```python
from build123d import *

# Parameters (mm, degrees)
BOSS_EXTRUDE1_DEPTH = 3.175
CUT_EXTRUDE1_REACH  = 5.175


with BuildPart() as part:
    # Sketch1 → Boss-Extrude1 (new body)
    with BuildSketch(Plane(origin=(0, 0, 0), x_dir=(0, 0, -1), z_dir=(1, 0, 0))):
        Polygon((0, 0), (-837.664111915, 0), (-1066.8, -396.875), (-1066.8, -800.1), (0, -800.1), align=None)
    extrude(amount=BOSS_EXTRUDE1_DEPTH)

    # Sketch2 → Cut-Extrude1 (cut, up to next)
    with BuildSketch(Plane(origin=(3.175, 0, 0), x_dir=(0, 0, -1), z_dir=(1, 0, 0)), mode=Mode.PRIVATE) as cut_extrude1_sk1:
        Polygon((-101.6, -396.875), (-101.6, -101.6), (-698.5, -101.6), (-698.5, -698.5), (-101.6, -698.5), align=None)
    cut_extrude1_tool1 = extrude(cut_extrude1_sk1.sketch, amount=-CUT_EXTRUDE1_REACH, mode=Mode.PRIVATE) & part.part
    add(cut_extrude1_tool1.solids().sort_by_distance((3.175, -400.05, 400.05))[0], mode=Mode.SUBTRACT)


solid = part.part
```
Can you work these out from the model? Positions are in its coordinate system, mm. Round coordinates to 2 decimals unless told otherwise and drop trailing zeros. Loops run counter-clockwise (first coordinate to the right, second up) from the corner with the lowest first, then second, coordinate; pieces in that order, holes last. Notation, with made-up numbers: M 76,24 L 118,24 A16 cw 118,40 Z; hole C 18.25,6.5 d9. An arc over 180 degrees is marked long. Answer in a Markdown table with one row per item.
1. Please list where these lines run through material, in increasing order: line 1 (Y direction, x = 0.2, z = 199); line 2 (Z direction, x = 0.45, y = -675); line 3 (Z direction, x = 2.55, y = -376). Write a range as from..to.
Established:
| item | result |
|---|---|
| line 1 | -800.1..-698.5, -101.6..0 |
| line 2 | 0..101.6, 698.5..1066.8 |
| line 3 | 0..101.6, 698.5..1054.75 |
2. If we section it at A-A, the plane z = 181: Please give me the cut outline in (x, y) (3 decimals), plus the area to 3 significant figures.
Established:
| item | result |
|---|---|
| outline | M 0,-800.1 L 3.175,-800.1 L 3.175,-698.5 L 0,-698.5 Z; M 0,-101.6 L 3.175,-101.6 L 3.175,0 L 0,0 Z |
| area | 645 mm² |
3. If we section it at D-D, the plane y = -88: Please give me the cut outline in (x, z) (3 decimals), plus the area to 3 significant figures.
Established:
| item | result |
|---|---|
| outline | M 0,0 L 3.175,0 L 3.175,888.471 L 0,888.471 Z |
| area | 2,820 mm² |
4. I'm going to push flat-ended pins straight in: pin 1 Ø1 at (x, y) = (1.5, -376.5) entering from +Z; pin 2 Ø1.5 at (x, y) = (1.5, -217) entering from +Z; pin 3 Ø1 at (x, z) = (1.5, 338) entering from +Y. Where does each tip first touch, or does it pass through?
Established:
| item | result |
|---|---|
| pin 1 | z = 1055.33 |
| pin 2 | z = 963.38 |
| pin 3 | y = 0 |
5. If we section it at B-B, the plane y = -460.5: Please give me the cut outline in (x, z) (3 decimals).
Established:
| item | result |
|---|---|
| outline | M 0,0 L 3.175,0 L 3.175,101.6 L 0,101.6 Z; M 0,698.5 L 3.175,698.5 L 3.175,1066.8 L 0,1066.8 Z |
6. If we section it at C-C, the plane x = 2.4: Please give me the cut outline in (y, z) (3 decimals).
Established:
| item | result |
|---|---|
| outline | M -800.1,0 L 0,0 L 0,837.664 L -396.875,1066.8 L -800.1,1066.8 Z; hole M -698.5,101.6 L -101.6,101.6 L -101.6,698.5 L -698.5,698.5 Z |
